Geometry: see drawing. Coordinates: mm, zero at the bounding-box minimum. A direction names the side the tool comes from. Coordinates: 2 decimals unless noted, no trailing zeros. Loops run counter-clockwise (first coordinate to the right, second up) from the corner with the lowest first, then second, coordinate; pieces in that order, holes last. Notation, with made-up numbers: (-26, 84) - (3, 84) arc R15 cw to (3, 101) - close; hole circle Ø4 at (10.25, 28). An arc over 180 degrees is marked (long way). Use one line per item in the form item = value.
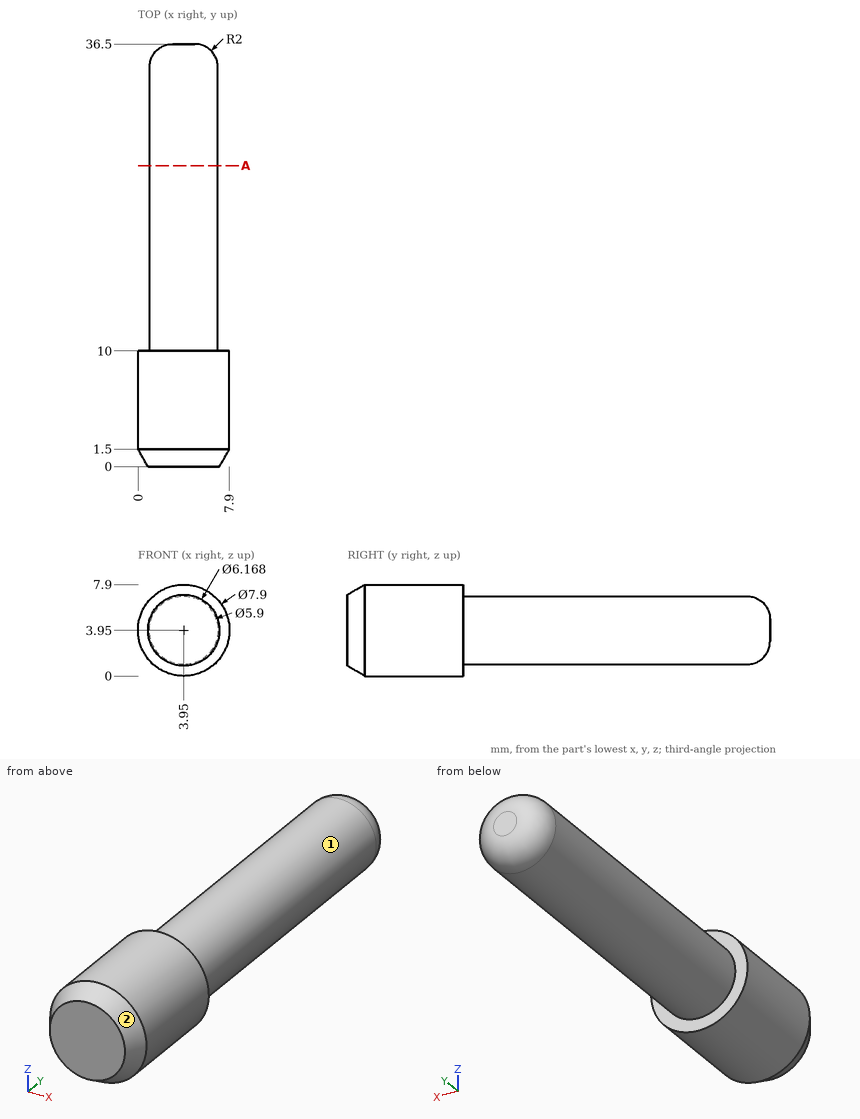
Q1. Set-up query: the marked faces 1 and 2. Return all of +Z, -Z, +X, -X, +Y, -Y with unobstructed straight access to the full face (end or side cutting, diameter ignored); none if empty.
Check values:
face_1 = +Y
face_2 = -Y
Q2. Cut plane A-A, the plane y = 26. Return loops of the section in (x, z).
Check values:
outline = circle Ø5.9 at (3.95, 3.95)
Q3. Ray query, line 1 along Z through (x, y) = (4, 20); line 2 along Y through (x, z) = (1.5, 1.5); line 3 along Y through (x, z) = (4.25, 7.5). Return the intervals inside material, ascending. Write a range as [from, to].
Check values:
line_1 = [1, 6.9]
line_2 = [0.66, 10]
line_3 = [0.83, 10]
Q4. First-contact query: P1, Ø3, axis at x = 3, y = 15, coming from the +Z side; P2, Ø1, axis at x = 1.5, y = 25.5, coming from the +Z side. Flat tips, straight axial feed; report the tip coordinate or a pass-through.
Check values:
P1 = 6.9
P2 = 6.16
